Part model, mm, in its own coordinate system. Face numbers are marked on the shaded views. A direction names the side the tool comes from. Give positions to 0.01 mm unless a question says otherwise; leave off trailing zeros. Write each loop counter-clockwise with the first axis right and the second up, starting at its lowest first coordinate (ties: lowest second). Pieces come first, ordered by that corner, then holes. Notation, with made-up numbers: M 50,75.5 L 76,75.5 A15 ccw 76,93.5 Z; hole C 44.5,48 d6. An arc over 180 degrees is marked long. Use CSV: the item, a comma, the result in double quotes. Start each with the question number.
Item 1: Which spindle directions (+Z, -Z, +X, -X, +Y, -Y) get a long thin tool onto all of the face, cutting with end or side? Do the marked faces 1 and 2. Say none if no direction does.
Item 2: Drill centre lines: line 1 (Y direction, x = -12, z = 24); line 2 (Y direction, x = -20, z = 26.5); line 3 (Z direction, x = -4, y = 28). Where is each one in solid material? Low to high. Write a range as [from, to].
Item 3: Pin check, flat tips, straight feed: pin 1 (1 mm diameter, centred on x = -1, z = 11, fed in from +Y); pin 2 (2 mm diameter, centred on x = -3.5, z = 12, fed in from -Y); pin 3 (8 mm diameter, centred on y = 18.5, z = 7.5, fed in from +X); pin 4 (1.8 mm diameter, centred on y = 13.5, z = 13, fed in from -X). Stop position of each tip, or through.
Item 4: Cut at B-B (y = 22.5). List the corners of the cut face in (x, z), then the cut area to 3 significant figures.
Item 5: Cut at A-A (x = -21.5). Count the separate pieces of the cut face and the enclosed holes in it, then the cut area to 3 significant figures.
Item 6: Mould opens along Y. For the marked faces 3, 4, 5 and 6 say: released by +Y, released by -Y, zero draft, split by the parting line, or undercut.
from build123d import *

# Parameters (mm, degrees)
BOSS_EXTRUDE1_DEPTH     = 45
CUT_EXTRUDE1_DEPTH      = 66.041883154
CUT_EXTRUDE1_DEPTH_BACK = 66.041883154
SKETCH2_R               = 13.7
CUT_EXTRUDE2_DEPTH      = 65.974294466
SKETCH4_W               = 5
SKETCH4_H               = 25
CUT_EXTRUDE3_DEPTH      = 15
CUT_EXTRUDE4_DEPTH      = 18
CUT_EXTRUDE5_DEPTH      = 3
SKETCH8_R               = 2.1
CUT_EXTRUDE6_DEPTH      = 15
FILLET1_R               = 2
FILLET2_R               = 0.5


with BuildPart() as part:
    # Sketch1 → Boss-Extrude1 (new body)
    with BuildSketch(Plane(origin=(0, 0, 0), x_dir=(1, 0, 0), z_dir=(0, 1, 0))):
        Polygon((0, 0), (-31.171444325, 0), (-25, -35), (0, -35), align=None)
    extrude(amount=BOSS_EXTRUDE1_DEPTH)

    # Sketch2 → Cut-Extrude1 (cut, two sides: drawn at the far end of the back side and taken through both)
    with BuildSketch(Plane(origin=(5.231510268, 0, 29.669369072), x_dir=(-0.9848077530122074, 0, 0.17364817766693474), z_dir=(-0.17364817766693474, 0, -0.9848077530122074)).offset(-CUT_EXTRUDE1_DEPTH_BACK)):
        with Locations((30.697880044, 22.5)):
            Circle(SKETCH2_R)
    extrude(amount=CUT_EXTRUDE1_DEPTH + CUT_EXTRUDE1_DEPTH_BACK, mode=Mode.SUBTRACT)

    # Sketch3 → Cut-Extrude2 (cut, through all)
    with BuildSketch(Plane.XY.offset(35)):
        Polygon((-5, 35), (-5, 40), (-10, 45), (0, 45), (0, 35), align=None)
        Polygon((-5, 10), (0, 10), (0, 0), (-10, 0), (-5, 5), align=None)
    extrude(amount=-CUT_EXTRUDE2_DEPTH, mode=Mode.SUBTRACT)

    # Sketch4 → Cut-Extrude3 (cut)
    with BuildSketch(Plane.XY.offset(35)):
        with Locations((-2.5, 22.5)):
            Rectangle(SKETCH4_W, SKETCH4_H)
    extrude(amount=-CUT_EXTRUDE3_DEPTH, mode=Mode.SUBTRACT)

    # Sketch5 → Cut-Extrude4 (cut)
    with BuildSketch(Plane.XY.offset(20)):
        Polygon((-5, 32.75), (-2.2, 32.75), (-2.2, 30), (0, 30), (0, 15), (-2.2, 15), (-2.2, 12.25), (-5, 12.25), align=None)
    extrude(amount=-CUT_EXTRUDE4_DEPTH, mode=Mode.SUBTRACT)

    # Sketch6 → Cut-Extrude5 (cut)
    with BuildSketch(Plane(origin=(-5, 0, 0), x_dir=(0, 0, -1), z_dir=(1, 0, 0))):
        with BuildLine():
            Line((-35, 19.5), (-35, 25.5))
            Line((-35, 25.5), (-34.25, 25.5))
            ThreePointArc((-34.25, 25.5), (-29.75, 22.5), (-34.25, 19.5))
            Line((-34.25, 19.5), (-35, 19.5))
        make_face()
    extrude(amount=-CUT_EXTRUDE5_DEPTH, mode=Mode.SUBTRACT)

    # Sketch8 → Cut-Extrude6 (cut)
    with BuildSketch(Plane(origin=(-30.231510268, 0, 5.330630928), x_dir=(0.17364817766693477, 0, 0.9848077530122074), z_dir=(-0.9848077530122072, 0, 0.17364817766693474))):
        with Locations((2.357101206, 40.2)):
            Circle(SKETCH8_R)
        with Locations((22.357101206, 40.2)):
            Circle(SKETCH8_R)
        with Locations((22.357101206, 4.8)):
            Circle(SKETCH8_R)
        with Locations((2.357101206, 4.8)):
            Circle(SKETCH8_R)
    extrude(amount=-CUT_EXTRUDE6_DEPTH, mode=Mode.SUBTRACT)

    # Fillet1
    fillet1_edges = [part.edges().sort_by_distance(p)[0] for p in [
        (-17.5, 45, 35),
        (-20.585722162, 0, 0),
        (-7.5, 2.5, 0),
        (-10, 0, 17.5),
        (-5, 7.5, 0),
        (-5, 5, 17.5),
        (-2.5, 10, 0),
        (-7.5, 2.5, 35),
        (-20.585722162, 45, 0),
        (-2.5, 35, 0),
        (-5, 37.5, 0),
        (-7.5, 42.5, 0),
        (-5, 40, 17.5),
        (-10, 45, 17.5),
        (-17.5, 0, 35),
        (-7.5, 42.5, 35),
    ]]
    fillet(fillet1_edges, radius=FILLET1_R)

    # Fillet2
    fillet2_edges = [part.edges().sort_by_distance(p)[0] for p in [
        (0, 22.5, 0),
        (0, 10, 11),
        (0, 35, 11),
        (0, 10.585786438, 0.585786438),
        (0, 34.414213562, 0.585786438),
        (-5, 35, 11),
        (-5, 10, 11),
        (-5, 31.335786438, 35),
        (-5, 38.216836977, 34.85841639),
        (-5, 6.783163023, 34.85841639),
        (-5.163269118, 39.963039656, 33.739113334),
        (-5.707902185, 34.292097815, 0.473407966),
        (-5.163269118, 5.036960344, 33.739113334),
        (-5.707902185, 10.707902185, 0.473407966),
        (0, 12.5, 20),
        (0, 32.5, 20),
        (-2.2, 30, 11),
        (0, 30, 11),
        (0, 15, 11),
        (-2.2, 15, 11),
        (-1.1, 15, 20),
        (-1.1, 30, 20),
        (-2.2, 31.375, 2),
        (-1.1, 30, 2),
        (0, 22.5, 2),
        (-1.1, 15, 2),
        (-2.2, 13.625, 2),
        (-5, 13.664213562, 35),
    ]]
    fillet(fillet2_edges, radius=FILLET2_R)


solid = part.part
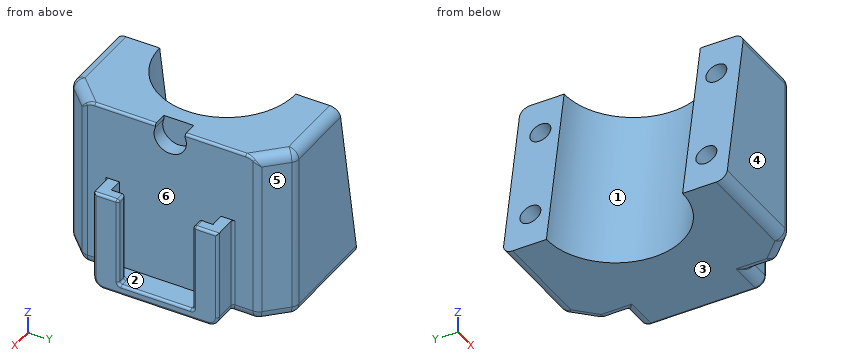
Worked answers:
1,face 1,"+Z, -X"
1,face 2,"+Z"
2,line 1,"y = [0, 2.86], [6.74, 38.26], [42.14, 45]"
2,line 2,"y = [0, 2.72], [6.88, 10.39], [34.61, 38.12], [42.28, 45]"
2,line 3,"z = [0, 2]"
3,pin 1,"stops at y = 35"
3,pin 2,"stops at y = 10"
3,pin 3,"stops at x = 0"
3,pin 4,"stops at x = -19.28"
4,outline,"M -17.26,0 L -0.5,0 A0.5 ccw 0,0.5 L 0,1.5 A0.5 ccw -0.5,2 L -5,2 L -5,29.75 L -8,29.75 L -8,35 L -11.09,35 Z"
4,area,"315 mm^2"
5,separate pieces,"2"
5,enclosed holes,"4"
5,area,"682 mm^2"
6,face 3,"zero draft"
6,face 4,"released by -Y"
6,face 5,"released by +Y"
6,face 6,"undercut"
